Study the drawing (mm; zero at the part's minimum x, y, z) and answer. Coordinates: 2 decimals unless noted, no trailing zeros. Order: outer loops, then holes, each group sorted by start corner. A loop starts at its lowest first (then second) coordinate and runs counter-clockwise, first axis right, second up. Notation, with made-up numbers: (42, 51) -> (90, 51) arc R18 cw to (90, 59) -> close; hole circle Ø11 at (37, 20). An arc over 180 degrees is marked (long way). Answer in a Markdown table with one row per item. Add a question column.
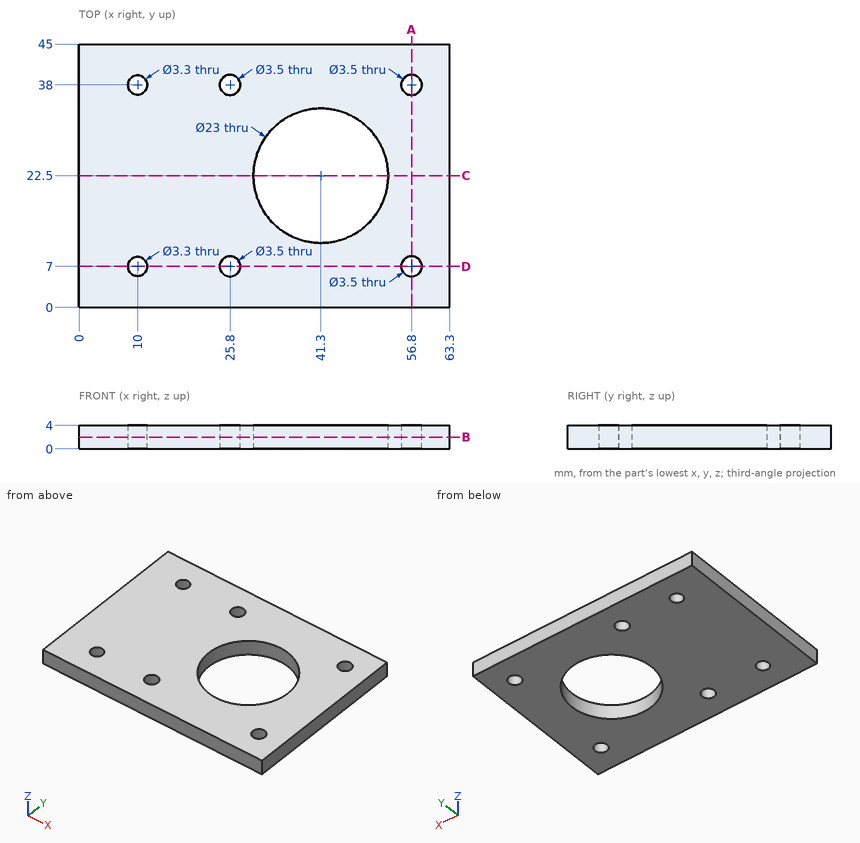
Q1. A cutting plane is placed at D-D (y = 7). Determine the outline of the cut face in (x, z).
Q2. Given pin 1 (5 mm diameter, centred on x = 34.5, y = 22.5, fed in from -Z), flat-ended and moving along its own axis, determine where the tip first touches the part or whether it passes through.
Q3. Straight lines are drawn through the part: line 1 (Y direction, x = 10, z = 0.85); line 2 (Y direction, x = 56.8, z = 1.9); line 3 (X direction, y = 38, z = 2.9). For each, find the intervals that lie inside material, in ascending order.
Q4. A cutting plane is placed at C-C (y = 22.5). Determine the outline of the cut face in (x, z), then the cut area to 3 significant figures.
Q5. A cutting plane is placed at A-A (x = 56.8). Determine the outline of the cut face in (y, z).
Q6. A cutting plane is placed at B-B (z = 2). Determine the outline of the cut face in (x, y), then the cut area to 3 significant figures.
Returned:
| question | item | result |
|---|---|---|
| 1 | outline | (0, 0) -> (8.35, 0) -> (8.35, 4) -> (0, 4) -> close; (11.65, 0) -> (24.05, 0) -> (24.05, 4) -> (11.65, 4) -> close; (27.55, 0) -> (55.05, 0) -> (55.05, 4) -> (27.55, 4) -> close; (58.55, 0) -> (63.3, 0) -> (63.3, 4) -> (58.55, 4) -> close |
| 2 | pin 1 | passes through |
| 3 | line 1 | y = 0 to 5.35, 8.65 to 36.35, 39.65 to 45 |
| 3 | line 2 | y = 0 to 5.25, 8.75 to 36.25, 39.75 to 45 |
| 3 | line 3 | x = 0 to 8.35, 11.65 to 24.05, 27.55 to 55.05, 58.55 to 63.3 |
| 4 | outline | (0, 0) -> (29.8, 0) -> (29.8, 4) -> (0, 4) -> close; (52.8, 0) -> (63.3, 0) -> (63.3, 4) -> (52.8, 4) -> close |
| 4 | area | 161 mm² |
| 5 | outline | (0, 0) -> (5.25, 0) -> (5.25, 4) -> (0, 4) -> close; (8.75, 0) -> (36.25, 0) -> (36.25, 4) -> (8.75, 4) -> close; (39.75, 0) -> (45, 0) -> (45, 4) -> (39.75, 4) -> close |
| 6 | outline | (0, 0) -> (63.3, 0) -> (63.3, 45) -> (0, 45) -> close; hole circle Ø3.3 at (10, 7); hole circle Ø3.3 at (10, 38); hole circle Ø3.5 at (25.8, 7); hole circle Ø3.5 at (25.8, 38); hole circle Ø23 at (41.3, 22.5); hole circle Ø3.5 at (56.8, 7); hole circle Ø3.5 at (56.8, 38) |
| 6 | area | 2,380 mm² |
